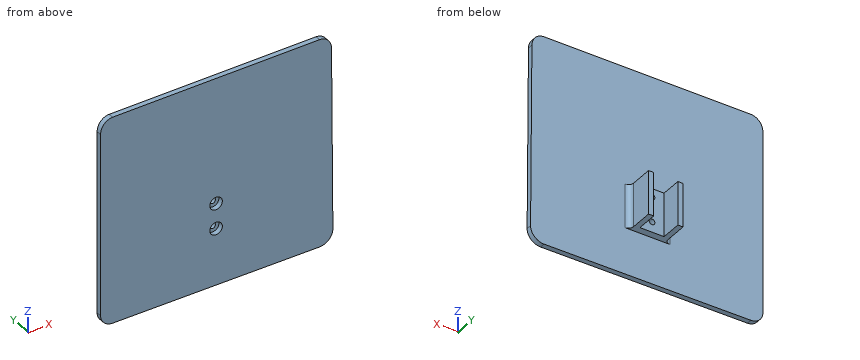
```python
from build123d import *

# Parameters (mm, degrees)
SKETCH1_R           = 1.655864604
BOSS_EXTRUDE1_DEPTH = 3
SKETCH2_W           = 20
SKETCH2_H           = 25.399582392
SKETCH2_R           = 1.655864604
BOSS_EXTRUDE2_DEPTH = 16
SKETCH3_W           = 14
SKETCH3_H           = 30.433665038
CUT_EXTRUDE1_DEPTH  = 12
FILLET1_R           = 3
SKETCH4_R           = 3.655864604
CUT_EXTRUDE2_DEPTH  = 3


with BuildPart() as part:
    # Sketch1 → Boss-Extrude1 (new body)
    with BuildSketch(Plane(origin=(0, 0, 0), x_dir=(1, 0, 0), z_dir=(0, 1, 0))):
        with BuildLine():
            Line((-67.62365194, 48.899661457), (-67.62365194, -56.801447555))
            add(Edge.make_bspline(
                [(-67.62365194, -56.801447555), (-67.62365194, -57.576529056), (-67.408945412, -59.103174242), (-66.539947264, -61.00790182), (-65.334097821, -62.438503957), (-64.120247313, -63.394550402), (-62.546848101, -64.127219326), (-61.250619214, -64.324861548), (-60.62365194, -64.324861548)],
                knots=[0, 0, 0, 0, 0.25, 0.5, 0.625, 0.75, 0.875, 1, 1, 1, 1], degree=3))
            Line((-60.62365194, -64.324861548), (59.37634806, -64.324861548))
            add(Edge.make_bspline(
                [(59.37634806, -64.324861548), (59.996985006, -64.324861548), (61.275308456, -64.133359368), (62.856831905, -63.405567156), (64.077573394, -62.44733485), (65.282373866, -61.023465146), (66.158364103, -59.118925072), (66.37634806, -57.580964506), (66.37634806, -56.801447555)],
                knots=[0, 0, 0, 0, 0.125, 0.25, 0.375, 0.5, 0.75, 1, 1, 1, 1], degree=3))
            Line((66.37634806, -56.801447555), (67.164580452, 48.899661457))
            ThreePointArc((67.164580452, 48.899661457), (64.882544637, 54.407688605), (59.373759242, 56.687893419))
            Line((59.373759242, 56.687893419), (-60.62365194, 55.899661457))
            ThreePointArc((-60.62365194, 55.899661457), (-65.573399408, 53.849408926), (-67.62365194, 48.899661457))
        make_face()
        with Locations((-0.62365194, 23.293074001)):
            Circle(SKETCH1_R, mode=Mode.SUBTRACT)
        with Locations((-0.62365194, 8.677667421)):
            Circle(SKETCH1_R, mode=Mode.SUBTRACT)
    extrude(amount=BOSS_EXTRUDE1_DEPTH)

    # Sketch2 → Boss-Extrude2 (add)
    with BuildSketch(Plane(origin=(0, 3, 0), x_dir=(1, 0, 0), z_dir=(0, 1, 0))):
        with Locations((-0.62365194, 16.648607969)):
            Rectangle(SKETCH2_W, SKETCH2_H)
        with Locations((-0.62365194, 8.677667421)):
            Circle(SKETCH2_R, mode=Mode.SUBTRACT)
        with Locations((-0.62365194, 23.293074001)):
            Circle(SKETCH2_R, mode=Mode.SUBTRACT)
    extrude(amount=BOSS_EXTRUDE2_DEPTH)

    # Sketch3 → Cut-Extrude1 (cut)
    with BuildSketch(Plane(origin=(0, 19, 0), x_dir=(1, 0, 0), z_dir=(0, 1, 0))):
        with Locations((-0.62365194, 16.661700324)):
            Rectangle(SKETCH3_W, SKETCH3_H)
    extrude(amount=-CUT_EXTRUDE1_DEPTH, mode=Mode.SUBTRACT)

    # Fillet1
    fillet1_edges = [part.edges().sort_by_distance(p)[0] for p in [
        (-10.62365194, 3, -16.648607969),
        (9.37634806, 3, -16.648607969),
    ]]
    fillet(fillet1_edges, radius=FILLET1_R)

    # Sketch4 → Cut-Extrude2 (cut)
    with BuildSketch(Plane.XZ):
        with Locations((-0.62365194, -8.677667421)):
            Circle(SKETCH4_R)
        with Locations((-0.62365194, -23.293074001)):
            Circle(SKETCH4_R)
    extrude(amount=-CUT_EXTRUDE2_DEPTH, mode=Mode.SUBTRACT)


solid = part.part
```
Verification items for the finished model (mm, model axes). Coordinates: 2 decimals unless noted, no trailing zeros. Loops run counter-clockwise (first coordinate to the right, second up) from the corner with the lowest first, then second, coordinate; pieces in that order, holes last. Notation, with made-up numbers: (21, 48.5) -> (61, 48.5) arc R6 ccw to (61, 53.5) -> close; hole circle Ø9 at (88.25, -8). An arc over 180 degrees is marked (long way). Answer in a Markdown table with one row per item.
1) Depth check by flat-ended pin: P1, Ø6.5, axis at x = -0.62, z = -23.29, coming from the -Y side; P2, Ø8, axis at x = -13, y = 4.5, coming from the -Z side; P3, Ø8, axis at x = 21, z = 6, coming from the +Y side; P4, Ø2.5, axis at x = -0.62, z = -8.68, coming from the +Y side. Enter the tip coordinate at first touch or a pass-through.
The answers:
| item | result |
|---|---|
| P1 | stops at y = 3 |
| P2 | stops at z = -56.24 |
| P3 | stops at y = 3 |
| P4 | passes through |
2) Section check B-B (x = 27). Record the cut outline in (y, z), and give its area (3 significant figures).
The answers:
| item | result |
|---|---|
| outline | (0, -56.48) -> (3, -56.48) -> (3, 64.32) -> (0, 64.32) -> close |
| area | 362 mm2 |
3) Section check C-C (z = 49). Record the cut outline in (x, y), and give its area (3 significant figures).
The answers:
| item | result |
|---|---|
| outline | (-67.62, 0) -> (66.43, 0) -> (66.43, 3) -> (-67.62, 3) -> close |
| area | 402 mm2 |
4) Scan lines: line 1 along X through (y, z) = (8, -28.5); line 2 along Y through (x, z) = (-29, 58); line 3 along Z through (x, y) = (2, 6). Record each from-to range of solid material in increasing order. Write a range as from..to.
The answers:
| item | result |
|---|---|
| line 1 | x = -10.62..-7.62, 6.38..9.38 |
| line 2 | y = 0..3 |
| line 3 | z = -29.35..-3.95 |
5) Section check A-A (y = 17.5). Record the cut outline in (x, z).
The answers:
| item | result |
|---|---|
| outline | (-10.62, -29.35) -> (-7.62, -29.35) -> (-7.62, -3.95) -> (-10.62, -3.95) -> close; (6.38, -29.35) -> (9.38, -29.35) -> (9.38, -3.95) -> (6.38, -3.95) -> close |
